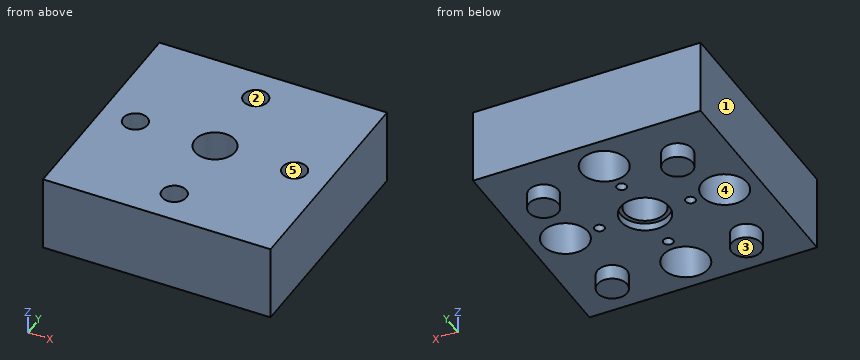
from build123d import *

# Parameters (mm, degrees)
SKETCH1_W           = 30
SKETCH1_H           = 30
BOSS_EXTRUDE1_DEPTH = 30
SKETCH2_R           = 0.65
CUT_EXTRUDE1_DEPTH  = 7
SKETCH3_R           = 1.95
BOSS_EXTRUDE2_DEPTH = 2
SKETCH4_R           = 3.2
SKETCH4_R_2         = 2.5
CUT_EXTRUDE2_DEPTH  = 1
SKETCH5_R           = 2.65
CUT_EXTRUDE3_DEPTH  = 46
SKETCH6_W           = 20
SKETCH6_H           = 32.666349305
CUT_EXTRUDE4_DEPTH  = 38.603191354
SKETCH7_R           = 3
CUT_EXTRUDE5_DEPTH  = 5
SKETCH8_R           = 1.6
CUT_EXTRUDE6_DEPTH  = 35.263683398


with BuildPart() as part:
    # Sketch1 → Boss-Extrude1 (new body)
    with BuildSketch(Plane(origin=(0, 0, 0), x_dir=(0, 0, -1), z_dir=(1, 0, 0))):
        Rectangle(SKETCH1_W, SKETCH1_H)
    extrude(amount=BOSS_EXTRUDE1_DEPTH)

    # Sketch2 → Cut-Extrude1 (cut)
    with BuildSketch(Plane(origin=(0, 0, -15), x_dir=(-1, 0, 0), z_dir=(0, 0, -1))):
        with Locations(Location((-15, 6.000101914, 0), (0, 0, 90))):
            Circle(SKETCH2_R)
        with Locations(Location((-21.001003121, 0.002997762, 0), (0, 0, 90))):
            Circle(SKETCH2_R)
        with Locations(Location((-8.997324254, 0.002997762, 0), (0, 0, 90))):
            Circle(SKETCH2_R)
        with Locations(Location((-15, -6.000101914, 0), (0, 0, 90))):
            Circle(SKETCH2_R)
    extrude(amount=-CUT_EXTRUDE1_DEPTH, mode=Mode.SUBTRACT)

    # Sketch3 → Boss-Extrude2 (add)
    with BuildSketch(Plane(origin=(0, 0, -15), x_dir=(-1, 0, 0), z_dir=(0, 0, -1))):
        with Locations(Location((-6.16, 8.84, 0), (0, 0, 270))):
            Circle(SKETCH3_R)
        with Locations(Location((-23.84, 8.84, 0), (0, 0, 270))):
            Circle(SKETCH3_R)
        with Locations(Location((-23.84, -8.84, 0), (0, 0, 270))):
            Circle(SKETCH3_R)
        with Locations(Location((-6.16, -8.84, 0), (0, 0, 270))):
            Circle(SKETCH3_R)
    extrude(amount=BOSS_EXTRUDE2_DEPTH)

    # Sketch4 → Cut-Extrude2 (cut)
    with BuildSketch(Plane(origin=(0, 0, -15), x_dir=(-1, 0, 0), z_dir=(0, 0, -1))):
        with Locations(Location((-15, 0, 0), (0, 0, 90))):
            Circle(SKETCH4_R)
        with Locations(Location((-15, 0, 0), (0, 0, 90))):
            Circle(SKETCH4_R_2, mode=Mode.SUBTRACT)
    extrude(amount=-CUT_EXTRUDE2_DEPTH, mode=Mode.SUBTRACT)

    # Sketch5 → Cut-Extrude3 (cut, through all)
    with BuildSketch(Plane(origin=(0, 0, -15), x_dir=(-1, 0, 0), z_dir=(0, 0, -1))):
        with Locations(Location((-15, 0, 0), (0, 0, 90))):
            Circle(SKETCH5_R)
    extrude(amount=-CUT_EXTRUDE3_DEPTH, mode=Mode.SUBTRACT)

    # Sketch6 → Cut-Extrude4 (cut, through all)
    with BuildSketch(Plane(origin=(30, 0, 0), x_dir=(0, 0, -1), z_dir=(1, 0, 0))):
        with Locations((-5, -1.333174652)):
            Rectangle(SKETCH6_W, SKETCH6_H)
    extrude(amount=-CUT_EXTRUDE4_DEPTH, mode=Mode.SUBTRACT)

    # Sketch7 → Cut-Extrude5 (cut)
    with BuildSketch(Plane(origin=(0, 0, -15), x_dir=(-1, 0, 0), z_dir=(0, 0, -1))):
        with Locations(Location((-15, 10.5, 0), (0, 0, 90))):
            Circle(SKETCH7_R)
        with Locations(Location((-15, -10.5, 0), (0, 0, 90))):
            Circle(SKETCH7_R)
        with Locations(Location((-25.5, 0, 0), (0, 0, 90))):
            Circle(SKETCH7_R)
        with Locations(Location((-4.5, 0, 0), (0, 0, 90))):
            Circle(SKETCH7_R)
    extrude(amount=-CUT_EXTRUDE5_DEPTH, mode=Mode.SUBTRACT)

    # Sketch8 → Cut-Extrude6 (cut, through all)
    with BuildSketch(Plane(origin=(0, 0, -10), x_dir=(-1, 0, 0), z_dir=(0, 0, -1))):
        with Locations(Location((-4.5, 0, 0), (0, 0, 90))):
            Circle(SKETCH8_R)
        with Locations(Location((-15, -10.5, 0), (0, 0, 90))):
            Circle(SKETCH8_R)
        with Locations(Location((-15, 10.5, 0), (0, 0, 90))):
            Circle(SKETCH8_R)
        with Locations(Location((-25.5, 0, 0), (0, 0, 90))):
            Circle(SKETCH8_R)
    extrude(amount=-CUT_EXTRUDE6_DEPTH, mode=Mode.SUBTRACT)


solid = part.part
Could you check a few things on this model? Use its own coordinates, in mm. Face numbers are marked on the shaded views. A direction names the side the tool comes from. Round coordinates to 2 decimals unless told otherwise and drop trailing zeros. Order: outer loops, then holes, each group sorted by start corner. A loop starts at its lowest first (then second) coordinate and runs counter-clockwise, first axis right, second up.
(1) Please list where these lines run through material, in increasing order: line 1 along X through (y, z) = (0, -11); line 2 along Y through (x, z) = (15.25, -12.75); line 3 along Z through (x, y) = (11.75, -1).
Response values:
line 1: x = 0 to 1.5, 7.5 to 8.35, 9.65 to 12.35, 17.65 to 20.35, 21.65 to 22.5, 28.5 to 30
line 2: y = -15 to -13.49, -7.51 to -6.6, -5.4 to -2.64, 2.64 to 5.4, 6.6 to 7.51, 13.49 to 15
line 3: z = -15 to -5
(2) I'm going to push flat-ended pins straight in: pin 1 (6.5 mm diameter, centred on x = 5, y = -1, fed in from -Z); pin 2 (8 mm diameter, centred on x = 22, y = -8, fed in from -Z); pin 3 (1.2 mm diameter, centred on x = 15, y = -6, fed in from -Z); pin 4 (5 mm diameter, centred on x = 15, y = 0, fed in from -Z). Where does each tip first touch, or does it pass through?
Response values:
pin 1: stops at z = -15
pin 2: stops at z = -17
pin 3: stops at z = -8
pin 4: passes through
(3) Imagine slicing it at B-B (y = 9.5). Write out the boundary of the cut face in (x, z), plus the area to 3 significant figures.
Response values:
outline: (0, -15) - (4.33, -15) - (4.33, -17) - (7.99, -17) - (7.99, -15) - (12.17, -15) - (12.17, -10) - (13.75, -10) - (13.75, -5) - (0, -5) - close; (16.25, -10) - (17.83, -10) - (17.83, -15) - (22.01, -15) - (22.01, -17) - (25.67, -17) - (25.67, -15) - (30, -15) - (30, -5) - (16.25, -5) - close
area: 274 mm2
(4) If we mould it in two halves opening along X, with no side actions, what happens to the marked faces 1, 2 and 3? For each: released by +X, released by -X, zero draft, split by the parting line, or undercut.
Response values:
face 1: released by -X
face 2: undercut
face 3: zero draft
(5) Imagine slicing it at C-C (y = 0). Count the separate pieces of the cut face and the enclosed holes in it, plus the area to 3 significant figures.
Response values:
separate pieces: 4
enclosed holes: 0
area: 136 mm2
(6) Imagine slicing it at A-A (z = -7). Write out the boundary of the cut face in (x, y), plus the area to 3 significant figures.
Response values:
outline: (0, -15) - (30, -15) - (30, 15) - (0, 15) - close; hole circle Ø3.2 at (4.5, 0); hole circle Ø5.3 at (15, 0); hole circle Ø3.2 at (15, -10.5); hole circle Ø3.2 at (15, 10.5); hole circle Ø3.2 at (25.5, 0)
area: 846 mm2
(7) Which directions (+Z, -Z, +X, -X, +Y, -Y) give clear straight access to the entire face, cutting with the end or side of a thin tool? Please do the marked faces 4 and 5.
Response values:
face 4: -Z
face 5: +Z, -Z
